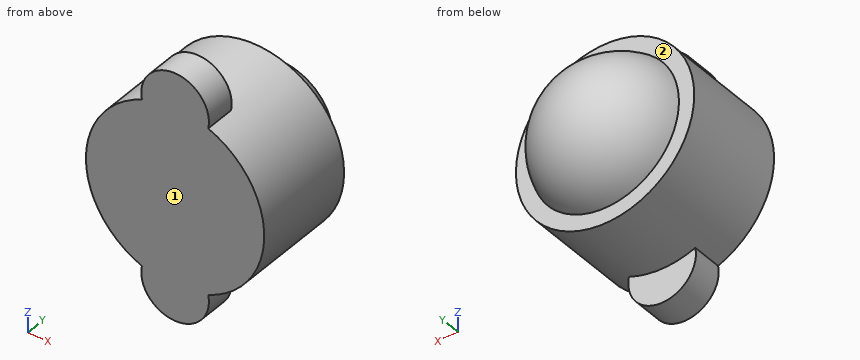
Autodesk Inventor part; units mm, degrees
ref_plane "Work Plane1" through (0, 7.112, 0) normal (0, -1, 0) x (1, 0, 0)
ref_plane "YZ Plane" through (0, 0, 0) normal (1, 0, 0) x (0, 1, 0)
ref_plane "XZ Plane" through (0, 0, 0) normal (0, 1, 0) x (-1, 0, 0)
sketch "Sketch1" plane through (0, 0, 0) normal (0, 1, 0) x (-1, 0, 0)
  circle A0 centre (0, 0) radius 7.366
  dimension "d0" = 14.732
extrude "Extrusion1" add sketch "Sketch1" along normal blind 8.89
ref_plane "Work Plane1" through (0, 7.112, 0) normal (0, -1, 0) x (1, 0, 0)
sketch "Sketch2" plane through (0, 7.112, 0) normal (0, -1, 0) x (1, 0, 0)
  arc A0 (-6.35, 0) -> (6.35, 0) centre (0, 0) ccw
  circle A1 centre (0, 0) radius 7.366 construction
  line L0 (-7.366, 0) -> (7.366, 0) construction
  line L1 (-6.35, 0) -> (6.35, 0)
  dimension "d4" = 12.7
revolve "Revolution1" add sketch "Sketch2" angle 360 about axis through (-7.366, 7.112, 0) along (1, 0, 0)
sketch "Sketch3" plane through (0, 0, 0) normal (0, -1, 0) x (1, 0, 0)
  line L0 (0, 7.3938) -> (0, -7.366) construction
  circle A0 centre (0, 0) radius 7.366 construction
  circle A1 centre (0, 7.3938) radius 2.794
  circle A2 centre (0, -7.366) radius 2.794
  dimension "d6" = 5.588
  dimension "d7" = 5.588
extrude "Extrusion2" add sketch "Sketch3" against normal blind 2.54
properties part number "caster ball 1 2 inch"
Can you work these out from the model? Positions are in its coordinate system, mm. Face numbers are marked on the shaded views. A direction names the side the tool comes from. Coordinates: 2 decimals unless noted, no trailing zeros. Loops run counter-clockwise (first coordinate to the right, second up) from the corner with the lowest first, then second, coordinate; pieces in that order, holes last. Notation, with made-up numbers: (23.5, 45) -> (60.5, 45) arc R22 cw to (60.5, 65) -> close; hole circle Ø6 at (64.5, 6.5). An arc over 180 degrees is marked (long way). Answer as a JSON object with one key per item and string values.
1) For the marked faces 1 and 2, which set-ups out of +Z, -Z, +X, -X, +Y, -Y let a thin tool reach every point of the face, with its end or its side?
Results:
{"face 1": "+Z, -Z, +X, -X, -Y", "face 2": "+Y"}
2) Imagine slicing it at A-A (x = 0). Please give me the cut outline in (y, z), then the cut area to 3 significant figures.
Results:
{"outline": "(0, -10.16) -> (2.54, -10.16) -> (2.54, -7.37) -> (8.89, -7.37) -> (8.89, -6.1) arc R6.35 ccw to (8.89, 6.1) -> (8.89, 7.37) -> (2.54, 7.37) -> (2.54, 10.19) -> (0, 10.19) -> close", "area": "186 mm^2"}
3) Imagine slicing it at B-B (z = 0). Please give me the cut outline in (x, y).
Results:
{"outline": "(-7.37, 0) -> (7.37, 0) -> (7.37, 8.89) -> (6.1, 8.89) arc R6.35 ccw to (-6.1, 8.89) -> (-7.37, 8.89) -> close"}
4) Imagine slicing it at D-D (x = -5.5). Please give me the cut outline in (y, z), then the cut area to 3 significant figures.
Results:
{"outline": "(0, -4.9) -> (8.89, -4.9) -> (8.89, -2.63) arc R3.17 ccw to (8.89, 2.63) -> (8.89, 4.9) -> (0, 4.9) -> close", "area": "92.3 mm^2"}
5) For P1, Ø8, axis at x = -3.5, z = 1, coming from the +Y side; P2, Ø1, axis at x = -3, z = 7, coming from the +Y side; P3, Ø3, axis at x = -3.5, y = 2.5, coming from the +Z side; P4, Ø1.5, axis at x = 4.5, z = 7, coming from the +Y side, each with a flat end and sliding along its axis, tell me the tip position at first contact or that it passes through.
Results:
{"P1": "stops at y = 13.46", "P2": "stops at y = 8.89", "P3": "stops at z = 9.34", "P4": "passes through"}
6) If I drill on line 1 (Z direction, x = 0, y = 8.5); line 2 (Y direction, x = -3.5, z = -6); line 3 (Z direction, x = -6, y = 8.5), over which ranges is the centre line in solid material (lowest first)?
Results:
{"line 1": "z = -7.37 to 7.37", "line 2": "y = 0 to 8.89", "line 3": "z = -4.27 to 4.27"}
7) Imagine slicing it at C-C (y = 5.25). Please give me the cut outline in (x, z), then the cut area to 3 significant figures.
Results:
{"outline": "circle Ø14.73 at (0, 0)", "area": "170 mm^2"}
